Source: CAD feature listing. Evaluate the final solid. Frame: model axes, mm. A direction names the side the tool comes from. Give positions to 0.01 mm unless a question says otherwise; leave off trailing zeros. Write each loop counter-clockwise with the first axis right and the second up, starting at its lowest first coordinate (ties: lowest second). Pieces come first, ordered by that corner, then holes. Notation, with made-up numbers: M -7.75,-17.75 L 43.25,-17.75 A20 cw 43.25,-3.75 Z; hole C 63,-14.5 d7. An arc over 180 degrees is marked long. Answer as a JSON object with one key per item and string values. Group by question number.
```python
from build123d import *

# Parameters (mm, degrees)
CYLINDER_R     = 1.5
CYLINDER_DEPTH = 10


with BuildPart() as cylinder:
    # Cylinder → Cylinder (new body)
    with BuildSketch(Plane.XY):
        Circle(CYLINDER_R)
    extrude(amount=CYLINDER_DEPTH)


with BuildPart() as ball_and_screw:
    # Sphere → Sphere (revolve)
    with BuildSketch(Plane.XZ):
        with BuildLine():
            ThreePointArc((0, -3), (3, 0), (0, 3))
            Line((0, 3), (0, -3))
        make_face()
    revolve(axis=Axis((0, 0, 0), (0, 0, 1)))

    # Fusion005: union Cylinder
    add(cylinder.part)


with BuildPart() as ball_and_screw_1:
    # Fusion005 placement: moved
    add(ball_and_screw.part.moved(Location((0, 0, -1))))


solid = ball_and_screw_1.part
```
(1) Section B-B, the plane y = 0. Return loops of the section in (x, z), plus the area to 3 significant figures.
(2) Contact query for flat-ended pins moving along their axis: pin 1 Ø3 at (x, z) = (-1.5, 6.5) entering from +Y; pin 2 Ø2 at (y, z) = (0, 5) entering from +X; pin 3 Ø2 at (x, z) = (-1.5, 6) entering from +Y. Output: stop coordinate, or through.
(3) Ray query, L1, parallel to Y at x = 0.05, z = 6.5; L2, parallel to Z at x = 0.35, y = 0.35. Return the intervals inside material, ascending. Write a range as [from, to].
(4) Section A-A, the plane z = 6.5. Return loops of the section in (x, y), plus the area to 3 significant figures.
(5) Access query for faces 1 (the cylindrical face through (-1.5, 0.07, 5.25)), 2 (the flat face through (0, 0, 9)). Directions: +Z, -Z, +X, -X, +Y, -Y. A direction counts if a zero-diameter tool reaches every point of the face in a straight line with its end or side. Return the directions, or none.
(6) Section D-D, the plane z = 0.5. Return loops of the section in (x, y), plus the area to 3 significant figures.
Reported:
{
 "1": {"outline": "M -1.5,1.6 A3 ccw long 1.5,1.6 L 1.5,9 L -1.5,9 Z", "area": "49.7 mm2"},
 "2": {"pin 1": "stops at y = 1.5", "pin 2": "stops at x = 1.5", "pin 3": "stops at y = 1.41"},
 "3": {"L1": "y = [-1.5, 1.5]", "L2": "z = [-3.96, 9]"},
 "4": {"outline": "C 0,0 d3", "area": "7.07 mm2"},
 "5": {"face 1": "+Z", "face 2": "+Z, +X, -X, +Y, -Y"},
 "6": {"outline": "C 0,0 d5.2", "area": "21.2 mm2"}
}
